```python
from build123d import *

# Parameters (mm, degrees)
F1_DEPTH = 152.4
F2_W     = 101.6
F2_H     = 76.2
F3_DEPTH = 76.2
F5_DEPTH = 76.2
F8_D     = 12.7
F9_D     = 6.35


with BuildPart() as f1:
    # F0 (on Front) → F1 (new body)
    with BuildSketch(Plane.XZ):
        Polygon((0, 98.280699), (-50.8, 98.280699), (-50.8, -104.919301), (101.6, -104.919301), (101.6, -54.119301), (0, -54.119301), align=None)
    extrude(amount=F1_DEPTH)

    # F2 (on face) → F3 (join)
    with BuildSketch(Plane.XY.offset(-54.119301)):
        with Locations((50.8, -38.1)):
            Rectangle(F2_W, F2_H)
    extrude(amount=F3_DEPTH)

    # F4 (on face) → F5 (cut)
    with BuildSketch(Plane.XZ.offset(76.2)):
        Polygon((101.6, 22.080699), (0, 22.080699), (101.6, -54.119301), align=None)
    extrude(amount=-F5_DEPTH, mode=Mode.SUBTRACT)

    # F8 (through all)
    with Locations(Plane.YZ):
        with Locations((-114.3, 60.180699)):
            Hole(F8_D / 2)

    # F9 (through all)
    with Locations(Plane.XY.offset(-54.119301)):
        with Locations((63.5, -114.3)):
            Hole(F9_D / 2)


solid = f1.part
```
Here's how the part is built. I have some questions about the finished solid (model axes, mm). A direction names the side the tool comes from. Round coordinates to 2 decimals unless told otherwise and drop trailing zeros. Order: outer loops, then holes, each group sorted by start corner. A loop starts at its lowest first (then second) coordinate and runs counter-clockwise, first axis right, second up. Notation, with made-up numbers: M -18.75,30.5 L 36.25,30.5 A19 cw 36.25,57.5 Z; hole C 82,10.25 d5. An arc over 180 degrees is marked long. One line per question, with ' | ' between items.
1) For pin 1 Ø10 at (y, z) = (-114.3, 60.18) entering from -X; pin 2 Ø2 at (x, y) = (10, -23.5) entering from +Z; pin 3 Ø10 at (x, y) = (35, -116) entering from +Z; pin 4 Ø1.5 at (y, z) = (-75, 66.5) entering from +X, each with a flat end and sliding along its axis, tell me the tip position at first contact or that it passes through.
Working result:
pin 1: through | pin 2: z = 15.33 | pin 3: z = -54.12 | pin 4: x = 0
2) I need wall thicknesses on line 1 along Z through (x, y) = (-30, -114); line 2 along Y through (x, z) = (63, -90); line 3 along Y through (x, z) = (63.5, -78.5) (3 decimals). Which ranges of each line are inside material? Lowest first, please.
Working result:
line 1: -104.92 to 53.84, 66.52 to 98.28 | line 2: -152.4 to -117.44, -111.16 to 0 | line 3: -152.4 to -117.475, -111.125 to 0
3) For faces 1 (the face through (39, -76.2, -25)), 2 (the face through (24, -75, -104.919)), which set-ups out of +Z, -Z, +X, -X, +Y, -Y let a thin tool reach every point of the face, with its end or its side?
Working result:
face 1: +Z, +X, -Y | face 2: -Z, +X, -X, +Y, -Y
4) If we mould it in two halves opening along Y, with no side actions, what happens to faces 3 (the face through (-25.76, -109.62, 64.47)), 4 (the face through (7, 0, -24)), 5 (the face through (-50.8, -75, -2))? For each: +Y half, -Y half, draft (parallel to the pull), parting line (faces both ways), or undercut.
Working result:
face 3: undercut | face 4: +Y half | face 5: draft
5) I want a section at D-D, the plane x = 39.5. Write out the boundary of the cut face in (y, z), then the cut area to 3 significant figures.
Working result:
outline: M -152.4,-104.92 L 0,-104.92 L 0,-7.54 L -76.2,-7.54 L -76.2,-54.12 L -152.4,-54.12 Z | area: 11,300 mm²
6) I want a section at B-B, the plane x = 63.5. Write out the boundary of the cut face in (y, z) (3 decimals).
Working result:
outline: M -152.4,-104.919 L -117.475,-104.919 L -117.475,-54.119 L -152.4,-54.119 Z; M -111.125,-104.919 L 0,-104.919 L 0,-25.544 L -76.2,-25.544 L -76.2,-54.119 L -111.125,-54.119 Z
7) I want a section at C-C, the plane y = -83.5. Write out the boundary of the cut face in (x, z).
Working result:
outline: M -50.8,-104.92 L 101.6,-104.92 L 101.6,-54.12 L 0,-54.12 L 0,98.28 L -50.8,98.28 Z
8) I want a section at A-A, the plane y = -114.3. Write out the boundary of the cut face in (x, z) (3 decimals).
Working result:
outline: M -50.8,-104.919 L 60.325,-104.919 L 60.325,-54.119 L 0,-54.119 L 0,53.831 L -50.8,53.831 Z; M -50.8,66.531 L 0,66.531 L 0,98.281 L -50.8,98.281 Z; M 66.675,-104.919 L 101.6,-104.919 L 101.6,-54.119 L 66.675,-54.119 Z
